Check sheet for the modelled part. Datum: model origin and axes. Units: mm. A direction names the side the tool comes from. Round coordinates to 2 decimals unless told otherwise and drop trailing zeros. Order: outer loops, then holes, each group sorted by start corner. A loop starts at its lowest first (then second) coordinate and runs counter-clockwise, first axis right, second up. Notation, with made-up numbers: (45, -38.75) -> (95, -38.75) arc R4 ccw to (95, -31.75) -> close; hole circle Ø5 at (-22, 60.25). An arc over 180 degrees is marked (long way). Answer in a Markdown table with one row per item. Add a question column.
1. Sectioned sample at B-B, the plane y = 77. Record the boundary of the cut face in (x, z).
2. Material ranges on L1, parallel to Z at x = -4.7, y = 101.5; L2, parallel to Y at x = -5.1, z = -86.25; L3, parallel to Z at x = -3.9, y = 101.5, recorded low to high. Write a range as from..to.
3. Draft check along Z on faces 4 (the flat face through (-6, 113.5, -48)), 5 (the flat face through (0, 57, -98.55)), 6 (the flat face through (-6, 60, -4.25)), 7 (the flat face through (-5, 6.5, -48)). Enter one of: +Z half, -Z half, draft (parallel to the pull), parting line (faces both ways), or undercut.
4. Sectioned sample at A-A, the plane x = 2.5. Record the boundary of the cut face in (y, z), then the cut area to 3 significant figures.
5. Depth check by flat-ended pin: P1, Ø1.5, axis at x = -6.5, y = 47.5, coming from the +Z side; P2, Ø1.3, axis at y = 71.5, z = -8.25, coming from the +X side; P3, Ø1.5, axis at x = -6, z = -36, coming from the +Y side; P4, Ø0.6, axis at x = -3.5, z = -55, coming from the +Y side. Enter the tip coordinate at first touch or a pass-through.
6. Access from +Z, -Z, +X, -X, +Y, -Y to the whole of each face (thin tool, end or side, straight path). Record for faces 1 (the flat face through (0, 0, 0)), 2 (the flat face through (-6, 60, -90.25)), 3 (the flat face through (-2.25, 61, -47)).
7. Sectioned sample at C-C, the plane z = -61. Record the boundary of the cut face in (x, y), then the cut area to 3 significant figures.
```python
from build123d import *

# Parameters (mm, degrees)
SKETCH1_W             = 8.5
SKETCH1_H             = 115
BOSS_EXTRUDE1_DEPTH   = 8.5
BOSS_EXTRUDE2_DEPTH   = 2
SKETCH3_W             = 8.3
SKETCH3_H             = 115
BOSS_EXTRUDE3_DEPTH   = 6.5
SKETCH4_W             = 86
SKETCH4_H             = 107
BOSS_EXTRUDE4_DEPTH   = 3
SKETCH5_W             = 78
SKETCH5_H             = 99
CUT_EXTRUDE1_DEPTH    = 152.589420805
FILLET2_R             = 3
FILLET12_R            = 2
FILLET13_R            = 2
SKETCH64_W            = 78
SKETCH64_H            = 99
BOSS_EXTRUDE12_DEPTH  = 5
M2X0_4_TAPPED_HOLE1_D = 1.6


with BuildPart() as part:
    # Sketch1 → Boss-Extrude1 (new body)
    with BuildSketch(Plane(origin=(4.25, 0, 0), x_dir=(0, 0, -1), z_dir=(1, 0, 0))):
        with Locations((0, 57.5)):
            Rectangle(SKETCH1_W, SKETCH1_H)
    extrude(amount=-BOSS_EXTRUDE1_DEPTH)

    # Sketch2 → Boss-Extrude2 (add)
    with BuildSketch(Plane(origin=(-4.25, 0, 0), x_dir=(0, -1, 0), z_dir=(-1, 0, 0))):
        Polygon((-6.5, -90.25), (-6.5, -4.25), (-114, -4.25), (-114, -98.55), (0, -98.55), (0, -90.25), align=None)
    extrude(amount=-BOSS_EXTRUDE2_DEPTH)

    # Sketch3 → Boss-Extrude3 (add)
    with BuildSketch(Plane(origin=(-2.25, 0, 0), x_dir=(0, 0, -1), z_dir=(1, 0, 0))):
        with Locations((94.4, 57.5)):
            Rectangle(SKETCH3_W, SKETCH3_H)
    extrude(amount=BOSS_EXTRUDE3_DEPTH)

    # Sketch4 → Boss-Extrude4 (add)
    with BuildSketch(Plane.ZY.offset(4.25)):
        with Locations((-47.25, 60)):
            Rectangle(SKETCH4_W, SKETCH4_H)
    extrude(amount=BOSS_EXTRUDE4_DEPTH)

    # Sketch5 → Cut-Extrude1 (cut, through all)
    with BuildSketch(Plane(origin=(-2.25, 0, 0), x_dir=(0, 0, -1), z_dir=(1, 0, 0))):
        with Locations((47.25, 60)):
            Rectangle(SKETCH5_W, SKETCH5_H)
    extrude(amount=-CUT_EXTRUDE1_DEPTH, mode=Mode.SUBTRACT)

    # Fillet2
    fillet2_edges = [part.edges().sort_by_distance(p)[0] for p in [
        (-4.75, 10.5, -8.25),
        (-4.75, 109.5, -8.25),
        (-4.75, 109.5, -86.25),
        (-4.75, 10.5, -86.25),
    ]]
    fillet(fillet2_edges, radius=FILLET2_R)

    # Fillet12
    fillet12_edges = [part.edges().sort_by_distance(p)[0] for p in [
        (-5.75, 6.5, -90.25),
    ]]
    fillet(fillet12_edges, radius=FILLET12_R)

    # Fillet13
    fillet13_edges = [part.edges().sort_by_distance(p)[0] for p in [
        (-5.75, 6.5, -4.25),
    ]]
    fillet(fillet13_edges, radius=FILLET13_R)

    # Sketch64 → Boss-Extrude12 (add)
    with BuildSketch(Plane(origin=(-2.25, 0, 0), x_dir=(0, 0, -1), z_dir=(1, 0, 0))):
        with Locations((47.25, 60)):
            Rectangle(SKETCH64_W, SKETCH64_H)
    extrude(amount=-BOSS_EXTRUDE12_DEPTH)

    # M2x0.4 Tapped Hole1 (through all)
    with Locations(Plane.ZY.offset(7.25)):
        with Locations((-8.25, 11.5), (-8.25, 41.5), (-8.25, 71.5), (-8.25, 101.5), (-86.25, 11.5), (-86.25, 41.5), (-86.25, 71.5), (-86.25, 101.5)):
            Hole(M2X0_4_TAPPED_HOLE1_D / 2)


solid = part.part
```
Answer key:
| question | item | result |
|---|---|---|
| 1 | outline | (-7.25, -90.25) -> (-4.25, -90.25) -> (-4.25, -98.55) -> (4.25, -98.55) -> (4.25, -90.25) -> (-2.25, -90.25) -> (-2.25, -4.25) -> (4.25, -4.25) -> (4.25, 4.25) -> (-4.25, 4.25) -> (-4.25, -4.25) -> (-7.25, -4.25) -> close |
| 2 | L1 | z = -90.25..-87.05, -85.45..-9.05, -7.45..-4.25 |
| 2 | L2 | y = 6.5..10.7, 12.3..40.7, 42.3..70.7, 72.3..100.7, 102.3..113.5 |
| 2 | L3 | z = -98.55..-87.05, -85.45..-9.05, -7.45..4.25 |
| 3 | face 4 | draft |
| 3 | face 5 | -Z half |
| 3 | face 6 | +Z half |
| 3 | face 7 | undercut |
| 4 | outline | (0, -98.55) -> (115, -98.55) -> (115, -90.25) -> (0, -90.25) -> close; (0, -4.25) -> (115, -4.25) -> (115, 4.25) -> (0, 4.25) -> close |
| 4 | area | 1,930 mm² |
| 5 | P1 | stops at z = -4.25 |
| 5 | P2 | passes through |
| 5 | P3 | stops at y = 113.5 |
| 5 | P4 | stops at y = 114 |
| 6 | face 1 | +Z, -Z, +X, -X, -Y |
| 6 | face 2 | -Z, -X, +Y, -Y |
| 6 | face 3 | +X, +Y, -Y |
| 7 | outline | (-7.25, 6.5) -> (-2.25, 6.5) -> (-2.25, 114) -> (-4.25, 114) -> (-4.25, 113.5) -> (-7.25, 113.5) -> close |
| 7 | area | 536 mm² |
